CAD build for the part. Positions are in the model's coordinates, mm. A direction names the side the tool comes from. Give positions to 0.01 mm unless a question says otherwise; leave off trailing zeros. Write each loop counter-clockwise with the first axis right and the second up, starting at its lowest first coordinate (ties: lowest second). Pieces come first, ordered by that corner, then holes. Notation, with made-up numbers: (-26.5, -7.75) - (-3.5, -7.75) arc R26 ccw to (-3.5, 16.25) - close; hole circle Ø1 at (-1.75, 47). An arc over 180 degrees is marked (long way). Put each result on its own line as item: value. Start each with the question number.
1. Wall check: line 1 (Y direction, x = 7.5, z = 2); line 2 (X direction, y = 4, z = 15); line 3 (Z direction, x = 51.5, y = -20.5). Give the ranges that are in metal, low to high.
2. Cut at B-B on x = 57. List the corners of the cut face in (y, z) (3 decimals), and give its area (3 significant figures).
3. Drop flat-ended pins along their axis: pin 1 (2 mm diameter, centred on x = -120, z = 15.5, fed in from +Y) (3 decimals); pin 2 (10 mm diameter, centred on x = -69, y = 26, fed in from +Z); pin 3 (2 mm diameter, centred on x = 100.5, y = -33.5, fed in from +Z). Give the stop position or say it passes through.
4. Cut at C-C on y = -14. List the corners of the cut face in (x, z), and give its area (3 significant figures).
5. Cut at D-D on x = -36.5. List the corners of the cut face in (y, z) (3 decimals).
6. Cut at A-A on z = 23. List the corners of the cut face in (x, y) (3 decimals).
7. Mould opens along X. For faces 1 (the flat face through (-3, 5, 0)), 2 (the flat face through (-120.884, 4, 14)), 3 (the flat face through (-118.884, 4, 14)), 4 (the flat face through (1, 42.882, 6)) say: +X half, -X half, draft (parallel to the pull), parting line (faces both ways), or undercut.
8. Tool access for faces 5 (the flat face through (-3, -33.118, 6)), 6 (the flat face through (117.116, 4, 14)), 7 (the flat face through (1, 44.882, 6)): list every direction of +Z, -Z, +X, -X, +Y, -Y with a clear straight run to the whole face (end or side of a thin tool).
from build123d import *

# Parameters (mm, degrees)
SKETCH31_W                     = 240
SKETCH31_H                     = 80
BASE_FLANGE1_DEPTH             = 2
EDGE_FLANGE1_STRIP_W           = 9.4732
EDGE_FLANGE1_STRIP_H           = 2
EDGE_FLANGE1_STRIP_CUT_DEPTH   = 240
EDGE_FLANGE1_STRIP_2_W         = 9.4732
EDGE_FLANGE1_STRIP_2_H         = 2
EDGE_FLANGE1_STRIP_CUT_2_DEPTH = 240
EDGE_FLANGE1_DEPTH             = 240
EDGE_FLANGE1_BEND_DEPTH        = 240
EDGE_FLANGE2_START             = -32.381792537
EDGE_FLANGE2_DEPTH             = 74.5268
EDGE_FLANGE2_2_OUTLINE_W       = 2
EDGE_FLANGE2_2_OUTLINE_H       = 28
EDGE_FLANGE2_2_DEPTH           = 74.5268
SKETCH52_W                     = 26.086706926
SKETCH52_H                     = 9.115658902
CUT_EXTRUDE2_DEPTH             = 10
SKETCH53_W                     = 26.086706926
SKETCH53_H                     = 0.049167759
CUT_EXTRUDE3_DEPTH             = 10
SKETCH61_R                     = 1.5
CUT_EXTRUDE8_DEPTH             = 148.637805464
SKETCH62_R                     = 1.5
CUT_EXTRUDE9_DEPTH             = 148.637805464


# Read off the part's stored shape, not the designer's step: Edge-Flange2
# Sheet-metal steps are written as plain solids
with BuildPart() as part:
    # Sketch31 → Base-Flange1 (new body)
    with BuildSketch(Plane.XY):
        with Locations((-0.883917881, 4.881607463)):
            Rectangle(SKETCH31_W, SKETCH31_H)
    extrude(amount=-BASE_FLANGE1_DEPTH)

    # Edge-Flange1 strip (across the edge) → Edge-Flange1 strip cut (cut)
    with BuildSketch(Plane(origin=(119.116082119, 44.881607463, 0), x_dir=(0, -1, 0), z_dir=(-1, 0, 0))):
        with Locations((-2, -1)):
            Rectangle(EDGE_FLANGE1_STRIP_W, EDGE_FLANGE1_STRIP_H)
    extrude(amount=EDGE_FLANGE1_STRIP_CUT_DEPTH, mode=Mode.SUBTRACT)

    # Edge-Flange1 strip 2 (across the edge) → Edge-Flange1 strip cut 2 (cut)
    with BuildSketch(Plane(origin=(-120.883917881, -35.118392537, 0), x_dir=(0, 1, 0), z_dir=(1, 0, 0))):
        with Locations((-2, -1)):
            Rectangle(EDGE_FLANGE1_STRIP_2_W, EDGE_FLANGE1_STRIP_2_H)
    extrude(amount=EDGE_FLANGE1_STRIP_CUT_2_DEPTH, mode=Mode.SUBTRACT)

    # Edge-Flange1 section (across the edge) → Edge-Flange1 (add)
    with BuildSketch(Plane(origin=(119.116082119, 44.881607463, 0), x_dir=(0, -1, 0), z_dir=(-1, 0, 0))):
        with BuildLine():
            Line((0, 0.7366), (0, 11))
            Line((0, 11), (2, 11))
            Line((2, 11), (2, 0.7366))
            ThreePointArc((2, 0.7366), (2.215745145, 0.215745145), (2.7366, 0))
            Line((2.7366, 0), (2.7366, -2))
            ThreePointArc((2.7366, -2), (0.801531583, -1.198468417), (0, 0.7366))
        make_face()
    extrude(amount=EDGE_FLANGE1_DEPTH)

    # Edge-Flange1 section 2 (across the edge) → Edge-Flange1 bend (add)
    with BuildSketch(Plane(origin=(-120.883917881, -35.118392537, 0), x_dir=(0, 1, 0), z_dir=(1, 0, 0))):
        with BuildLine():
            Line((0, 0.7366), (0, 11))
            Line((0, 11), (2, 11))
            Line((2, 11), (2, 0.7366))
            ThreePointArc((2, 0.7366), (2.215745145, 0.215745145), (2.7366, 0))
            Line((2.7366, 0), (2.7366, -2))
            ThreePointArc((2.7366, -2), (0.801531583, -1.198468417), (0, 0.7366))
        make_face()
    extrude(amount=EDGE_FLANGE1_BEND_DEPTH)

    # Edge-Flange2 outline → Edge-Flange2 (cut)
    with BuildSketch(Plane(origin=(0, 0, 0), x_dir=(1, 0, 0), z_dir=(0, 1, 0)).offset(EDGE_FLANGE2_START)):
        with BuildLine():
            ThreePointArc((117.116082119, 2), (118.530295681, 1.414213562), (119.116082119, 0))
            Line((119.116082119, 0), (119.116082119, 2))
            Line((119.116082119, 2), (117.116082119, 2))
        make_face()
        with BuildLine():
            ThreePointArc((-120.883917881, 0), (-120.298131443, 1.414213562), (-118.883917881, 2))
            Line((-118.883917881, 2), (-120.883917881, 2))
            Line((-120.883917881, 2), (-120.883917881, 0))
        make_face()
    extrude(amount=EDGE_FLANGE2_DEPTH, mode=Mode.SUBTRACT)

    # Edge-Flange2 2 outline → Edge-Flange2 2 (add)
    with BuildSketch(Plane(origin=(0, 0, 0), x_dir=(1, 0, 0), z_dir=(0, 1, 0)).offset(EDGE_FLANGE2_START)):
        with Locations((118.116082119, -14)):
            Rectangle(EDGE_FLANGE2_2_OUTLINE_W, EDGE_FLANGE2_2_OUTLINE_H)
        with Locations((-119.883917881, -14)):
            Rectangle(EDGE_FLANGE2_2_OUTLINE_W, EDGE_FLANGE2_2_OUTLINE_H)
    extrude(amount=EDGE_FLANGE2_2_DEPTH)

    # Sketch52 → Cut-Extrude2 (cut)
    with BuildSketch(Plane(origin=(0, -33.118392537, 0), x_dir=(1, 0, 0), z_dir=(0, 1, 0))):
        with Locations((-65.439575559, -6.39300279)):
            Rectangle(SKETCH52_W, SKETCH52_H)
    cut_extrude2 = extrude(amount=-CUT_EXTRUDE2_DEPTH, mode=Mode.SUBTRACT)

    # Sketch53 → Cut-Extrude3 (cut)
    with BuildSketch(Plane(origin=(0, -33.118392537, 0), x_dir=(1, 0, 0), z_dir=(0, 1, 0))):
        with Locations((-65.439575559, -10.975416121)):
            Rectangle(SKETCH53_W, SKETCH53_H)
    cut_extrude3 = extrude(amount=-CUT_EXTRUDE3_DEPTH, mode=Mode.SUBTRACT)

    # Mirror3: Cut-Extrude3 across plane
    add(cut_extrude3.mirror(Plane(origin=(0, 0, 0), x_dir=(0, 0, 1), z_dir=(1, 0, 0))), mode=Mode.SUBTRACT)

    # Mirror4: Cut-Extrude2, Cut-Extrude3 across plane
    add(cut_extrude2.mirror(Plane(origin=(0, 0, 0), x_dir=(0, 0, 1), z_dir=(1, 0, 0))), mode=Mode.SUBTRACT)
    add(cut_extrude3.mirror(Plane(origin=(0, 0, 0), x_dir=(0, 0, 1), z_dir=(1, 0, 0))), mode=Mode.SUBTRACT)

    # Sketch61 → Cut-Extrude8 (cut, through all)
    with BuildSketch(Plane(origin=(0, 44.881607463, 0), x_dir=(1, 0, 0), z_dir=(0, 1, 0))):
        with Locations(Location((111.616082119, -5.4966, 0), (0, 0, 270))):
            Circle(SKETCH61_R)
    extrude(amount=-CUT_EXTRUDE8_DEPTH, mode=Mode.SUBTRACT)

    # Sketch62 → Cut-Extrude9 (cut, through all)
    with BuildSketch(Plane(origin=(0, 44.881607463, 0), x_dir=(1, 0, 0), z_dir=(0, 1, 0))):
        with Locations(Location((-113.383917881, -5.4966, 0), (0, 0, 270))):
            Circle(SKETCH62_R)
    extrude(amount=-CUT_EXTRUDE9_DEPTH, mode=Mode.SUBTRACT)


solid = part.part
Report:
1. line 1: y = -35.12 to -33.12, 42.88 to 44.88
1. line 2: x = -120.88 to -118.88, 117.12 to 119.12
1. line 3: z = -2 to 0
2. outline: (-35.118, 0.737) arc R2.737 ccw to (-32.382, -2) - (42.145, -2) arc R2.737 ccw to (44.882, 0.737) - (44.882, 11) - (42.882, 11) - (42.882, 0.737) arc R0.737 cw to (42.145, 0) - (-32.382, 0) arc R0.737 cw to (-33.118, 0.737) - (-33.118, 1.835) - (-35.118, 1.835) - close
2. area: 183 mm²
3. pin 1: stops at y = 42.145
3. pin 2: stops at z = 0
3. pin 3: stops at z = 11
4. outline: (-120.88, 0) arc R2 ccw to (-118.88, -2) - (117.12, -2) arc R2 ccw to (119.12, 0) - (119.12, 28) - (117.12, 28) - (117.12, 0) - (-118.88, 0) - (-118.88, 28) - (-120.88, 28) - close
4. area: 590 mm²
5. outline: (-35.118, 0.737) arc R2.737 ccw to (-32.382, -2) - (42.145, -2) arc R2.737 ccw to (44.882, 0.737) - (44.882, 11) - (42.882, 11) - (42.882, 0.737) arc R0.737 cw to (42.145, 0) - (-32.382, 0) arc R0.737 cw to (-33.118, 0.737) - (-33.118, 11) - (-35.118, 11) - close
6. outline: (-120.884, -32.382) - (-118.884, -32.382) - (-118.884, 42.145) - (-120.884, 42.145) - close; (117.116, -32.382) - (119.116, -32.382) - (119.116, 42.145) - (117.116, 42.145) - close
7. face 1: undercut
7. face 2: -X half
7. face 3: undercut
7. face 4: draft
8. face 5: +Z, +X, -X
8. face 6: +Z
8. face 7: +Z, -Z, +X, -X, +Y
